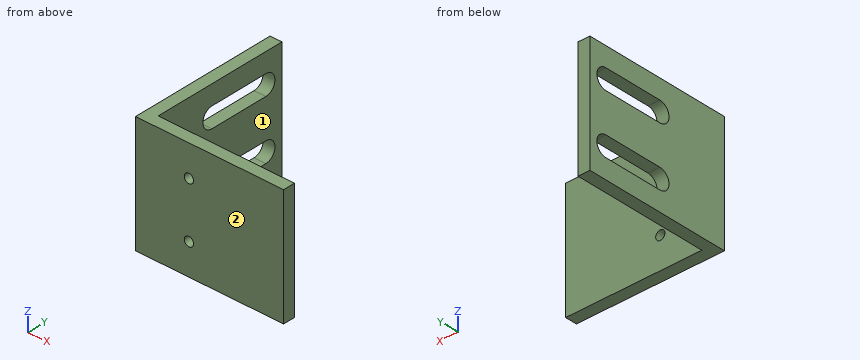
Autodesk Inventor part; units mm, degrees
ref_plane "YZ Plane" through (0, 0, 0) normal (1, 0, 0) x (0, 1, 0)
ref_plane "XZ Plane" through (0, 0, 0) normal (0, 1, 0) x (-1, 0, 0)
ref_plane "XY Plane" through (0, 0, 0) normal (0, 0, 1) x (1, 0, 0)
sketch "Skizze1" plane through (0, 0, 0) normal (0, 0, 1) x (1, 0, 0)
  line L0 (0, 0) -> (25, 0)
  line L1 (2, 2) -> (2, 25)
  line L2 (2, 25) -> (0, 25)
  line L3 (0, 25) -> (0, 0)
  line L4 (2, 2) -> (25, 2)
  line L5 (25, 2) -> (25, 0)
  dimension "d0" = 2
  dimension "d1" = 25
  dimension "d2" = 25
extrude "Extrusion1" add sketch "Skizze1" along normal blind 20
sketch "Skizze2" plane through (0, 0, 0) normal (0, -1, 0) x (1, 0, 0)
  line L0 (25, 20) -> (0, 20)
  line L1 (0, 0) -> (0, 20)
  line L2 (0, 0) -> (25, 0)
  line L3 (25, 0) -> (25, 20)
  line L4 (9, 20) -> (9, 0)
  line L5 (0, 10) -> (25, 10)
  point P0 (9, 14.7)
  point P1 (9, 5.3)
  dimension "d5" = 9
  dimension "d6" = 9.4
hole "Bohrung1" at (9, 0, 14.7) at (9, 0, 5.3) direction (0, 1, 0) diameter 1.567 end through all
sketch "Skizze3" plane through (2, 2, 0) normal (1, 0, 0) x (0, 0, -1)
  line L0 (0, 0) -> (-20, 0)
  line L1 (0, 23) -> (-20, 23)
  line L2 (-13.3, 20) -> (-13.3, 10)
  line L3 (-16.7, 10) -> (-16.7, 20)
  line L4 (-3.3, 20) -> (-3.3, 10)
  line L5 (-6.7, 10) -> (-6.7, 20)
  line L6 (-10, 23) -> (-10, 0)
  line L7 (-15, 20) -> (-15, 10)
  line L8 (-5, 10) -> (-5, 20)
  arc A0 (-13.3, 20) -> (-16.7, 20) centre (-15, 20) ccw
  arc A1 (-3.3, 20) -> (-6.7, 20) centre (-5, 20) ccw
  arc A2 (-6.7, 10) -> (-3.3, 10) centre (-5, 10) ccw
  arc A3 (-16.7, 10) -> (-13.3, 10) centre (-15, 10) ccw
  point P0 (0, -2)
  dimension "d14" = 10
  dimension "d15" = 3.4
  dimension "d16" = 3
  dimension "d18" = 10
extrude "Extrusion2" cut sketch "Skizze3" against normal through all
properties part number "13_0204_070"
Geometry check sheet. Reference: the model listing, model coordinates, mm. Face numbers are marked on the shaded views. A direction names the side the tool comes from. Give positions to 0.01 mm unless a question says otherwise; leave off trailing zeros. Order: outer loops, then holes, each group sorted by start corner. A loop starts at its lowest first (then second) coordinate and runs counter-clockwise, first axis right, second up. Notation, with made-up numbers: (-39, 39) - (-21, 39) arc R38 ccw to (-21, 77) - close; hole circle Ø6 at (-30, -33.5). An arc over 180 degrees is marked (long way). Write item = value, one per line. Start each with the question number.
1) Gauge pin test, flat ends, axial feed: pin 1 Ø1.4 at (x, z) = (9, 5.3) entering from +Y; pin 2 Ø6 at (x, z) = (19, 7) entering from +Y; pin 3 Ø10 at (y, z) = (18.5, 15) entering from +X. Record the tip position at first contact, or that the pin passes through.
2) Scan lines: L1, parallel to Z at x = 9, y = 1.5; L2, parallel to X at y = 1.55, z = 5.3; L3, parallel to X at y = 4.25, z = 3. Record each from-to range of solid material in increasing order.
3) Access from +Z, -Z, +X, -X, +Y, -Y to the whole of each face (thin tool, end or side, straight path). Record for the marked faces 1 and 2.
4) Section check A-A (x = 9). Enter the section's corners in (y, z), then the cut area to 3 significant figures.
5) Section check D-D (y = 8.5). Enter the section's corners in (x, z), then the cut area to 3 significant figures.
6) Section check C-C (z = 5). Enter the section's corners in (x, y).
7) Section check B-B (y = 18.25). Enter the section's corners in (x, z).
Geometry check:
q1.pin_1 = through
q1.pin_2 = 2
q1.pin_3 = 2
q2.L1 = 0 to 4.52, 6.08 to 13.92, 15.48 to 20
q2.L2 = 0 to 8.22, 9.78 to 25
q2.L3 = 0 to 2
q3.face_1 = +Z, -Z, +X, +Y
q3.face_2 = +Z, -Z, +X, -X, -Y
q4.outline = (0, 0) - (2, 0) - (2, 4.52) - (0, 4.52) - close; (0, 6.08) - (2, 6.08) - (2, 13.92) - (0, 13.92) - close; (0, 15.48) - (2, 15.48) - (2, 20) - (0, 20) - close
q4.area = 33.7 mm2
q5.outline = (0, 0) - (2, 0) - (2, 20) - (0, 20) - close
q5.area = 40.0 mm2
q6.outline = (0, 0) - (8.28, 0) - (8.28, 2) - (2, 2) - (2, 10.3) - (0, 10.3) - close; (0, 23.7) - (2, 23.7) - (2, 25) - (0, 25) - close; (9.72, 0) - (25, 0) - (25, 2) - (9.72, 2) - close
q7.outline = (0, 0) - (2, 0) - (2, 3.3) - (0, 3.3) - close; (0, 6.7) - (2, 6.7) - (2, 13.3) - (0, 13.3) - close; (0, 16.7) - (2, 16.7) - (2, 20) - (0, 20) - close
